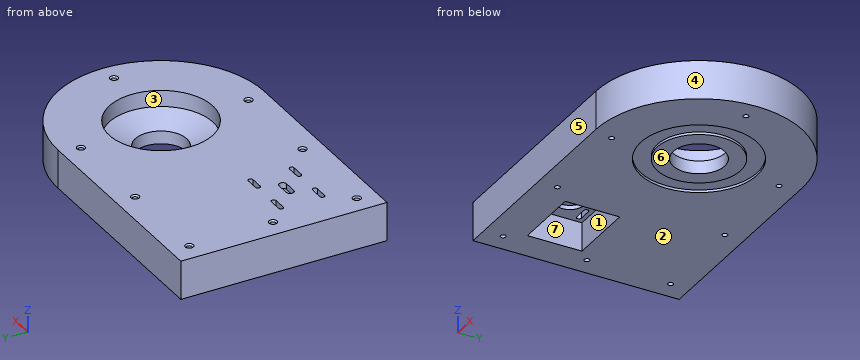
from build123d import *

# Parameters (mm, degrees)
SKETCH1_R                                       = 2.05
BOSS_EXTRUDE1_DEPTH                             = 15
CSK_FOR_M3_FLAT_HEAD_MACHINE_SCREW1_D           = 3.6
CSK_FOR_M3_FLAT_HEAD_MACHINE_SCREW1_CSINK_D     = 6.3
CSK_FOR_M3_FLAT_HEAD_MACHINE_SCREW1_CSINK_ANGLE = 90
CUT_EXTRUDE1_START                              = -10
SKETCH5_R                                       = 40.2
CUT_EXTRUDE1_DEPTH                              = 20
SKETCH6_R                                       = 20
CUT_EXTRUDE2_DEPTH                              = 191.26297592
CUT_EXTRUDE3_DEPTH                              = 22.27
M3_CLEARANCE_HOLE1_D                            = 3.6
M5_CLEARANCE_HOLE1_D                            = 5.8
CUT_EXTRUDE4_DEPTH                              = 3.27
CUT_EXTRUDE5_DEPTH                              = 190.1981842
SKETCH15_R                                      = 45.15
SKETCH15_R_2                                    = 32.35
CUT_EXTRUDE6_DEPTH                              = 2


with BuildPart() as part:
    # Sketch1 → Boss-Extrude1 (new, symmetric)
    with BuildSketch(Plane.XY):
        with BuildLine():
            Line((0, 80), (-170, 80))
            Line((-170, 80), (-170, -80))
            Line((-170, -80), (0, -80))
            ThreePointArc((0, -80), (80, 0), (0, 80))
        make_face()
        with Locations((-155, 65)):
            Circle(SKETCH1_R, mode=Mode.SUBTRACT)
        with Locations((-80, 65)):
            Circle(SKETCH1_R, mode=Mode.SUBTRACT)
        with Locations((-5, 65)):
            Circle(SKETCH1_R, mode=Mode.SUBTRACT)
        with Locations(Location((-155, -65, 0), (0, 0, 180))):
            Circle(SKETCH1_R, mode=Mode.SUBTRACT)
        with Locations(Location((-80, -65, 0), (0, 0, 180))):
            Circle(SKETCH1_R, mode=Mode.SUBTRACT)
        with Locations(Location((-5, -65, 0), (0, 0, 180))):
            Circle(SKETCH1_R, mode=Mode.SUBTRACT)
        with Locations(Location((-155, 0, 0), (0, 0, 180))):
            Circle(SKETCH1_R, mode=Mode.SUBTRACT)
        with Locations((65, 0)):
            Circle(SKETCH1_R, mode=Mode.SUBTRACT)
    extrude(amount=BOSS_EXTRUDE1_DEPTH, both=True)

    # CSK for M3 Flat Head Machine Screw1 (through all)
    with Locations(Plane.XY.offset(15)):
        with Locations((-5, -65), (-80, -65), (-155, -65), (-155, 0), (-155, 65), (-80, 65), (-5, 65), (65, 0)):
            CounterSinkHole(CSK_FOR_M3_FLAT_HEAD_MACHINE_SCREW1_D / 2, CSK_FOR_M3_FLAT_HEAD_MACHINE_SCREW1_CSINK_D / 2, counter_sink_angle=CSK_FOR_M3_FLAT_HEAD_MACHINE_SCREW1_CSINK_ANGLE)

    # Sketch5 → Cut-Extrude1 (cut)
    with BuildSketch(Plane(origin=(0, 0, -15), x_dir=(-1, 0, 0), z_dir=(0, 0, -1)).offset(CUT_EXTRUDE1_START)):
        Circle(SKETCH5_R)
    extrude(amount=-CUT_EXTRUDE1_DEPTH, mode=Mode.SUBTRACT)

    # Sketch6 → Cut-Extrude2 (cut, through all)
    with BuildSketch(Plane(origin=(0, 0, -15), x_dir=(-1, 0, 0), z_dir=(0, 0, -1))):
        Circle(SKETCH6_R)
    extrude(amount=-CUT_EXTRUDE2_DEPTH, mode=Mode.SUBTRACT)

    # Sketch7 → Cut-Extrude3 (cut)
    with BuildSketch(Plane(origin=(0, 0, -15), x_dir=(-1, 0, 0), z_dir=(0, 0, -1))):
        Polygon((103.85, -51.15), (146.15, -51.15), (146.15, -8.85), (103.85, -8.85), (93.85, -8.85), (93.85, -51.15), align=None)
    extrude(amount=-CUT_EXTRUDE3_DEPTH, mode=Mode.SUBTRACT)

    # M3 Clearance Hole1 (through all)
    with Locations(Plane(origin=(0, 0, 7.27), x_dir=(-1, 0, 0), z_dir=(0, 0, -1))):
        with Locations((109, -14), (141, -14), (141, -46), (109, -46), (99, -14), (99, -46), (131, -46), (131, -14)):
            Hole(M3_CLEARANCE_HOLE1_D / 2)

    # M5 Clearance Hole1 (through all)
    with Locations(Plane(origin=(0, 0, 7.27), x_dir=(-1, 0, 0), z_dir=(0, 0, -1))):
        with Locations((125, -30), (115, -30)):
            Hole(M5_CLEARANCE_HOLE1_D / 2)

    # Sketch13 → Cut-Extrude4 (cut)
    with BuildSketch(Plane(origin=(0, 0, 7.27), x_dir=(-1, 0, 0), z_dir=(0, 0, -1))):
        with BuildLine():
            Line((115, -18.85), (125, -18.85))
            ThreePointArc((125, -18.85), (136.15, -30), (125, -41.15))
            Line((125, -41.15), (115, -41.15))
            ThreePointArc((115, -41.15), (103.85, -30), (115, -18.85))
        make_face()
    extrude(amount=-CUT_EXTRUDE4_DEPTH, mode=Mode.SUBTRACT)

    # Sketch14 → Cut-Extrude5 (cut, through all)
    with BuildSketch(Plane(origin=(0, 0, 7.27), x_dir=(-1, 0, 0), z_dir=(0, 0, -1))):
        with BuildLine():
            Line((115, -27.1), (125, -27.1))
            ThreePointArc((125, -27.1), (127.9, -30), (125, -32.9))
            Line((125, -32.9), (115, -32.9))
            ThreePointArc((115, -32.9), (112.1, -30), (115, -27.1))
        make_face()
        with BuildLine():
            Line((99, -12.2), (109, -12.2))
            ThreePointArc((109, -12.2), (110.8, -14), (109, -15.8))
            Line((109, -15.8), (99, -15.8))
            ThreePointArc((99, -15.8), (97.2, -14), (99, -12.2))
        make_face()
        with BuildLine():
            Line((131, -12.2), (141, -12.2))
            ThreePointArc((141, -12.2), (142.8, -14), (141, -15.8))
            Line((141, -15.8), (131, -15.8))
            ThreePointArc((131, -15.8), (129.2, -14), (131, -12.2))
        make_face()
        with BuildLine():
            Line((141, -47.8), (131, -47.8))
            ThreePointArc((131, -47.8), (129.2, -46), (131, -44.2))
            Line((131, -44.2), (141, -44.2))
            ThreePointArc((141, -44.2), (142.8, -46), (141, -47.8))
        make_face()
        with BuildLine():
            Line((109, -47.8), (99, -47.8))
            ThreePointArc((99, -47.8), (97.2, -46), (99, -44.2))
            Line((99, -44.2), (109, -44.2))
            ThreePointArc((109, -44.2), (110.8, -46), (109, -47.8))
        make_face()
    extrude(amount=-CUT_EXTRUDE5_DEPTH, mode=Mode.SUBTRACT)

    # Sketch15 → Cut-Extrude6 (cut)
    with BuildSketch(Plane(origin=(0, 0, -15), x_dir=(-1, 0, 0), z_dir=(0, 0, -1))):
        Circle(SKETCH15_R)
        Circle(SKETCH15_R_2, mode=Mode.SUBTRACT)
    extrude(amount=-CUT_EXTRUDE6_DEPTH, mode=Mode.SUBTRACT)

    # Sketch16 → Revolve3 (revolve)
    with BuildSketch(Plane(origin=(0, 0, 0), x_dir=(1, 0, 0), z_dir=(0, 1, 0)), mode=Mode.PRIVATE) as revolve3_sk:
        Polygon((20, 5), (40.2, 5), (40.2, -2.352198732), align=None)
    revolve(revolve3_sk.sketch.rotate(Axis((0, 0, -9.069234204), (0, 0, 1)), 180), axis=Axis((0, 0, -9.069234204), (0, 0, 1)))


solid = part.part
Input: part model. Units: mm. Frame: model coordinates. Face numbers are marked on the shaded views. A direction names the side the tool comes from. Give positions to 0.01 mm unless a question says otherwise; leave off trailing zeros. Use one line per item in the form item = value. Start each with the question number.
1) Draft query along Y for the marked faces 4, 5, 6 and 7. Return one class per face: pulls with the +Y half, pulls with the -Y half, needs draft (parallel to the pull), parting line crosses it, or undercut.
2) Set-up query: the marked faces 1, 2 and 3. Return all of +Z, -Z, +X, -X, +Y, -Y with unobstructed straight access to the full face (end or side cutting, diameter ignored); none if empty.
3) Pin query (flat end, axial travel): pin 1 (4 mm diameter, centred on x = 45.5, z = 7, fed in from +Y); pin 2 (5.5 mm diameter, centred on x = -80, y = 65, fed in from +Z); pin 3 (3 mm diameter, centred on x = 33.5, y = 16.5, fed in from +Z). Return the tip coordinate at first contact, or that it passes through.
4) Ray query, probe 1 along Y at (x, z) = (-80, 3); probe 2 along X at (y, z) = (-65, -3.75); probe 3 along Y at (x, z) = (-155, -0.75). Return the intervals inside material, ascending. Write a range as from..to.
Outcome:
q1.face_4 = parting line crosses it
q1.face_5 = pulls with the -Y half
q1.face_6 = needs draft
q1.face_7 = undercut
q2.face_1 = -Z
q2.face_2 = -Z, +X, -X, +Y, -Y
q2.face_3 = +Z
q3.pin_1 = 67.14
q3.pin_2 = 14.6
q3.pin_3 = 1.86
q4.probe_1 = -80..-67.05, -62.95..62.95, 67.05..80
q4.probe_2 = -170..-157.05, -152.95..-82.05, -77.95..-7.05, -2.95..46.64
q4.probe_3 = -80..-67.05, -62.95..-2.05, 2.05..62.95, 67.05..80
